```python
from build123d import *

# Parameters (mm, degrees)
BOSS_EXTRUDE1_DEPTH      = 438.15
BOSS_EXTRUDE1_DEPTH_BACK = 57.15
SKETCH2_R                = 1.984375
CUT_EXTRUDE1_DEPTH       = 439.353336876
SKETCH3_R                = 1.984375
CUT_EXTRUDE2_DEPTH       = 439.353336876
CUT_EXTRUDE3_DEPTH       = 439.353336876
CUT_EXTRUDE3_DEPTH_BACK  = 439.353336876
SKETCH4_R                = 1.984375


with BuildPart() as part:
    # Sketch1 → Boss-Extrude1 (new, two sides: drawn at the far end of the back side and taken through both)
    with BuildSketch(Plane.XY.offset(-BOSS_EXTRUDE1_DEPTH_BACK)):
        Polygon((0, 0), (-8.980256121, 8.980256121), (-9.878281733, 8.082230509), (0, -1.796051224), (9.878281733, 8.082230509), (8.980256121, 8.980256121), align=None)
    extrude(amount=BOSS_EXTRUDE1_DEPTH + BOSS_EXTRUDE1_DEPTH_BACK)

    # Sketch2 → Cut-Extrude1 (cut, through all)
    with BuildSketch(Plane(origin=(0, 0, 0), x_dir=(0, 0, 1), z_dir=(-0.7071067811865469, 0.7071067811865481, 0))):
        with Locations(Location((431.8, 7.62, 0), (0, 0, 270))):
            Circle(SKETCH2_R)
        with Locations(Location((419.1, 7.62, 0), (0, 0, 270))):
            Circle(SKETCH2_R)
    extrude(amount=-CUT_EXTRUDE1_DEPTH, mode=Mode.SUBTRACT)

    # Sketch3 → Cut-Extrude2 (cut, through all)
    with BuildSketch(Plane(origin=(0, 0, 0), x_dir=(0, 0, -1), z_dir=(0.7071067811865483, 0.7071067811865468, 0))):
        with Locations(Location((-425.45, 7.62, 0), (0, 0, 90))):
            Circle(SKETCH3_R)
    extrude(amount=-CUT_EXTRUDE2_DEPTH, mode=Mode.SUBTRACT)

    # Sketch4 → Cut-Extrude3 (cut, two sides: drawn at the far end of the back side and taken through both)
    with BuildSketch(Plane(origin=(0, 0, 0), x_dir=(1, 0, 0), z_dir=(0, 1, 0)).offset(-CUT_EXTRUDE3_DEPTH_BACK)):
        with Locations(Location((0, 12.7, 0), (0, 0, 270))):
            Circle(SKETCH4_R)
    extrude(amount=CUT_EXTRUDE3_DEPTH + CUT_EXTRUDE3_DEPTH_BACK, mode=Mode.SUBTRACT)


solid = part.part
```
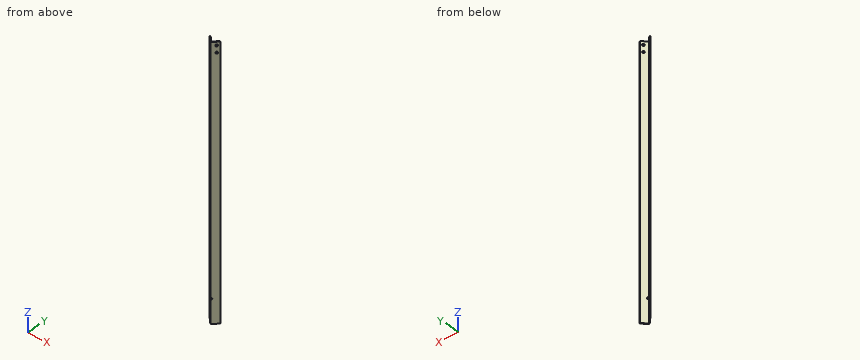
Work out the finished part from the listing and answer in its coordinate system (mm). Round coordinates to 2 decimals unless told otherwise and drop trailing zeros. Loops run counter-clockwise (first coordinate to the right, second up) from the corner with the lowest first, then second, coordinate; pieces in that order, holes last. Notation, with made-up numbers: (34.5, 59) -> (81.5, 59) arc R26 ccw to (81.5, 81) -> close; hole circle Ø8 at (4, 67.25). An arc over 180 degrees is marked (long way). Write each question's results on one line, items separated by ' | '. Start each with the question number.
1. Section A-A (z = 340) is taken. Determine the outline of the cut face in (x, y).
2. Given pin 1 Ø2.5 at (x, z) = (0, -12.7) entering from -Y; pin 2 Ø3 at (x, z) = (5.5, 225) entering from +Y; pin 3 Ø4 at (y, z) = (1, 335.5) entering from -X; pin 4 Ø2 at (y, z) = (3, 51) entering from -X, each flat-ended and moving along its own axis, determine where each tip first touches the part or whether it passes through.
3. Find the intervals of material crossed by probe 1 along Z at (x, y) = (0, -0.55); probe 2 along Z at (x, y) = (5.25, 4); probe 3 along X at (y, z) = (8.5, 127), in increasing order. Write a range as from..to.
Evaluation:
1) outline: (-9.88, 8.08) -> (0, -1.8) -> (9.88, 8.08) -> (8.98, 8.98) -> (0, 0) -> (-8.98, 8.98) -> close
2) pin 1: passes through | pin 2: stops at y = 7 | pin 3: stops at x = -4.8 | pin 4: stops at x = -5.8
3) probe 1: z = -57.15..-14.68, -10.72..438.15 | probe 2: z = -57.15..417.43, 420.77..430.13, 433.47..438.15 | probe 3: x = -9.46..-8.5, 8.5..9.46
